Input: part model. Units: mm. Frame: model coordinates. Face numbers are marked on the shaded views. A direction names the side the tool comes from. Coordinates: 2 decimals unless noted, no trailing zeros. Order: outer loops, then holes, each group sorted by start corner. A loop starts at its lowest first (then second) coordinate and runs counter-clockwise, first axis right, second up. Notation, with made-up numbers: (7.5, 52) - (56.5, 52) arc R17 cw to (56.5, 69) - close; hole circle Ø8 at (34.5, 27). An arc over 180 degrees is marked (long way). One line per question, with ' | ' between items.
from build123d import *

# Parameters (mm, degrees)
F0_W     = 19.05
F0_H     = 361.95
F1_DEPTH = 711.2


with BuildPart() as f1:
    # F0 (on Top) → F1 (new body)
    with BuildSketch(Plane.XY):
        Polygon((0, 381), (-19.05, 381), (-19.05, 0), (0, 0), (0, 361.95), align=None)
        Polygon((1143, 381), (0, 381), (0, 361.95), (1123.95, 361.95), (1143, 361.95), align=None)
        with Locations((1133.475, 180.975)):
            Rectangle(F0_W, F0_H)
        Polygon((1524, 0), (1143, 381), (1143, 361.95), (1504.95, 0), align=None)
    extrude(amount=F1_DEPTH)


solid = f1.part
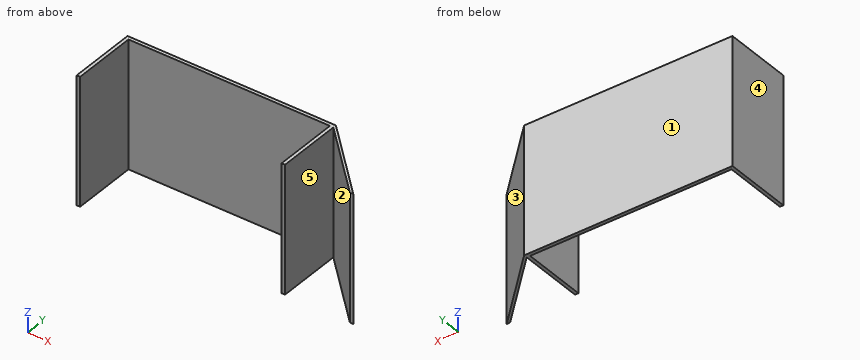
Item 1: Draft query along X for the marked faces 3, 4 and 5. Return one class per face: released by +X, released by -X, zero draft, split by the parting line, or undercut.
Data:
face 3: released by +X | face 4: released by -X | face 5: undercut
Item 2: Access query for the marked faces 1 and 2. Directions: +Z, -Z, +X, -X, +Y, -Y. A direction counts if a zero-diameter tool reaches every point of the face in a straight line with its end or side. Return the directions, or none.
Data:
face 1: +Z, -Z, +X, -X, +Y | face 2: +Z, -Z, -Y
Item 3: Section C-C on x = 634.5. Return the cut outline in (y, z), and give its area (3 significant figures).
Data:
outline: (361.95, 0) - (381, 0) - (381, 711.2) - (361.95, 711.2) - close | area: 13,500 mm^2
Item 4: Ray query, line 1 (X direction, y = 96, z = 657); line 2 (X direction, y = 182.5, z = 37); line 3 (Y direction, x = 776, z = 391.5). Return the intervals inside material, ascending.
Data:
line 1: -19.05 to 0, 1123.95 to 1143, 1408.95 to 1428 | line 2: -19.05 to 0, 1123.95 to 1143, 1322.45 to 1341.5 | line 3: 361.95 to 381
Item 5: Contact query for flat-ended pins moving along their axis: P1, Ø3, axis at y = 208, z = 158.5, coming from the +X side; P2, Ø3, axis at x = 684, z = 114.5, coming from the -Y side; P3, Ø10, axis at y = 67.5, z = 383, coming from the +X side. Output: stop coordinate, or through.
Data:
P1: x = 1317.5 | P2: y = 361.95 | P3: x = 1461.5
Item 6: Section B-B on z = 517. Return the cut outline in (x, y), and give its area (3 significant figures).
Data:
outline: (-19.05, 0) - (0, 0) - (0, 361.95) - (1123.95, 361.95) - (1123.95, 0) - (1143, 0) - (1143, 361.95) - (1504.95, 0) - (1524, 0) - (1143, 381) - (-19.05, 381) - close | area: 43,000 mm^2
Item 7: Section A-A on y = 60.5. Return the cut outline in (x, z).
Data:
outline: (-19.05, 0) - (0, 0) - (0, 711.2) - (-19.05, 711.2) - close; (1123.95, 0) - (1143, 0) - (1143, 711.2) - (1123.95, 711.2) - close; (1444.45, 0) - (1463.5, 0) - (1463.5, 711.2) - (1444.45, 711.2) - close
